Could you check a few things on this drawing? It's one solid part, dimensions in mm from its lowest x, y, z. Round coordinates to 2 decimals unless told otherwise and drop trailing zeros. Loops run counter-clockwise (first coordinate to the right, second up) from the corner with the lowest first, then second, coordinate; pieces in that order, holes last. Notation, with made-up numbers: (21.5, -2.75) -> (39.5, -2.75) arc R7 cw to (39.5, 10.25) -> close; hole circle Ø5 at (79, 4). An arc over 180 degrees is marked (long way). Put each result on its own line as item: value. Start each with the question number.
1. Imagine slicing it at D-D, the plane y = 25. Please give me the cut outline in (x, z).
2. Imagine slicing it at B-B, the plane x = 3.05. Please give me the cut outline in (y, z) (1 decimal), and give its area (3 significant figures).
3. Imagine slicing it at C-C, the plane y = 171.5. Please give me the cut outline in (x, z) (1 decimal).
4. I'm going to push flat-ended pins straight in: P1, Ø3, axis at x = 5, y = 104, coming from the +Z side; P2, Ø1.6, axis at x = 2.5, z = 300, coming from the +Y side. Where does each tip first touch, or does it pass through?
5. Imagine slicing it at A-A, the plane y = 129. Please give me the cut outline in (x, z) (1 decimal), and give its area (4 significant figures).
6. I need wall thicknesses on line 1 (Z direction, x = 4.3, y = 217) (1 decimal); line 2 (Z direction, x = 3.4, y = 179) (1 decimal); line 3 (Z direction, x = 3.2, y = 43). Which ranges of each line are inside material? Lowest first, please. Write a range as [from, to].
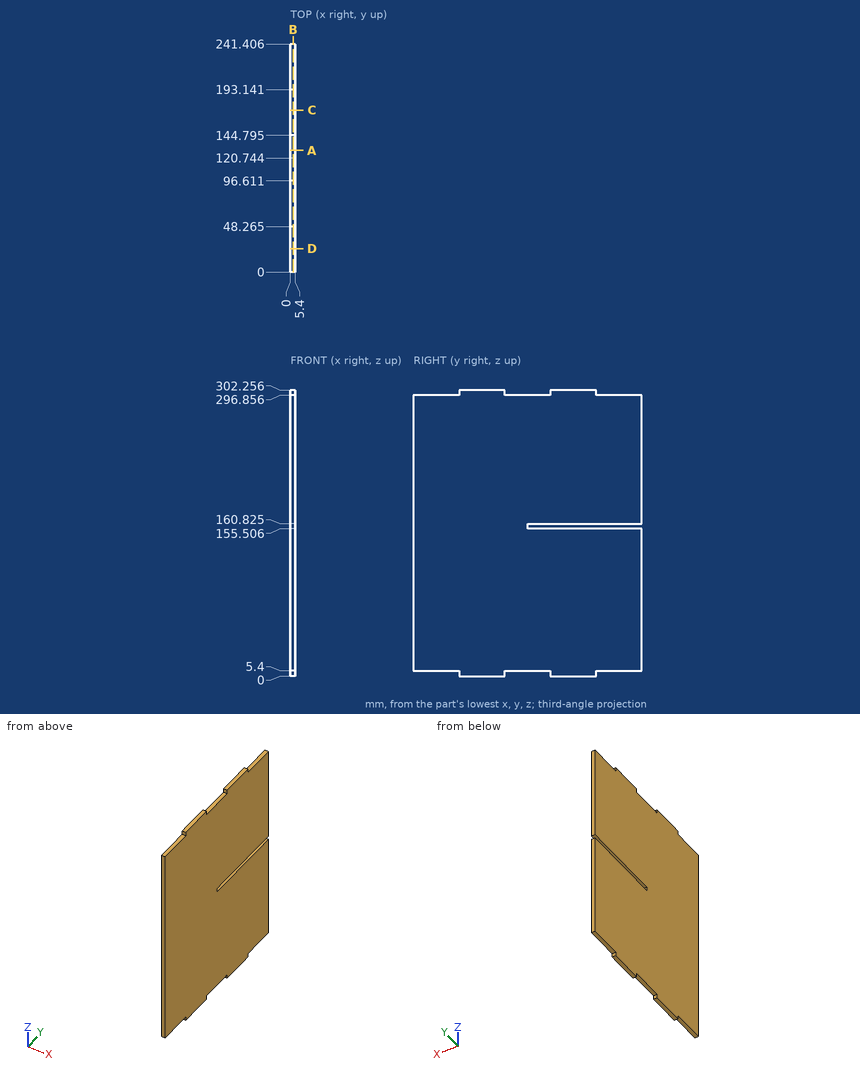
Entries:
1. outline: (0, 5.4) -> (5.4, 5.4) -> (5.4, 296.86) -> (0, 296.86) -> close
2. outline: (0, 5.4) -> (48.3, 5.4) -> (48.3, 0) -> (96.6, 0) -> (96.6, 5.4) -> (144.8, 5.4) -> (144.8, 0) -> (193.1, 0) -> (193.1, 5.4) -> (241.4, 5.4) -> (241.4, 155.5) -> (120.7, 155.5) -> (120.7, 160.8) -> (241.4, 160.8) -> (241.4, 296.9) -> (193.1, 296.9) -> (193.1, 302.3) -> (144.8, 302.3) -> (144.8, 296.9) -> (96.6, 296.9) -> (96.6, 302.3) -> (48.3, 302.3) -> (48.3, 296.9) -> (0, 296.9) -> close
2. area: 70,800 mm^2
3. outline: (0, 0) -> (5.4, 0) -> (5.4, 155.5) -> (0, 155.5) -> close; (0, 160.8) -> (5.4, 160.8) -> (5.4, 302.3) -> (0, 302.3) -> close
4. P1: z = 296.86
4. P2: y = 193.14
5. outline: (0, 5.4) -> (5.4, 5.4) -> (5.4, 155.5) -> (0, 155.5) -> close; (0, 160.8) -> (5.4, 160.8) -> (5.4, 296.9) -> (0, 296.9) -> close
5. area: 1,545 mm^2
6. line 1: [5.4, 155.5], [160.8, 296.9]
6. line 2: [0, 155.5], [160.8, 302.3]
6. line 3: [5.4, 296.86]
